Design review of the part shown in the three views and the two pictorial views. Dimensions are in mm from the part's minimum x, y and z. A direction names the side the tool comes from. Give positions to 0.01 mm unless a question says otherwise; leave off trailing zeros. Order: outer loops, then holes, each group sorted by start corner. A loop starts at its lowest first (then second) coordinate and runs counter-clockwise, first axis right, second up.
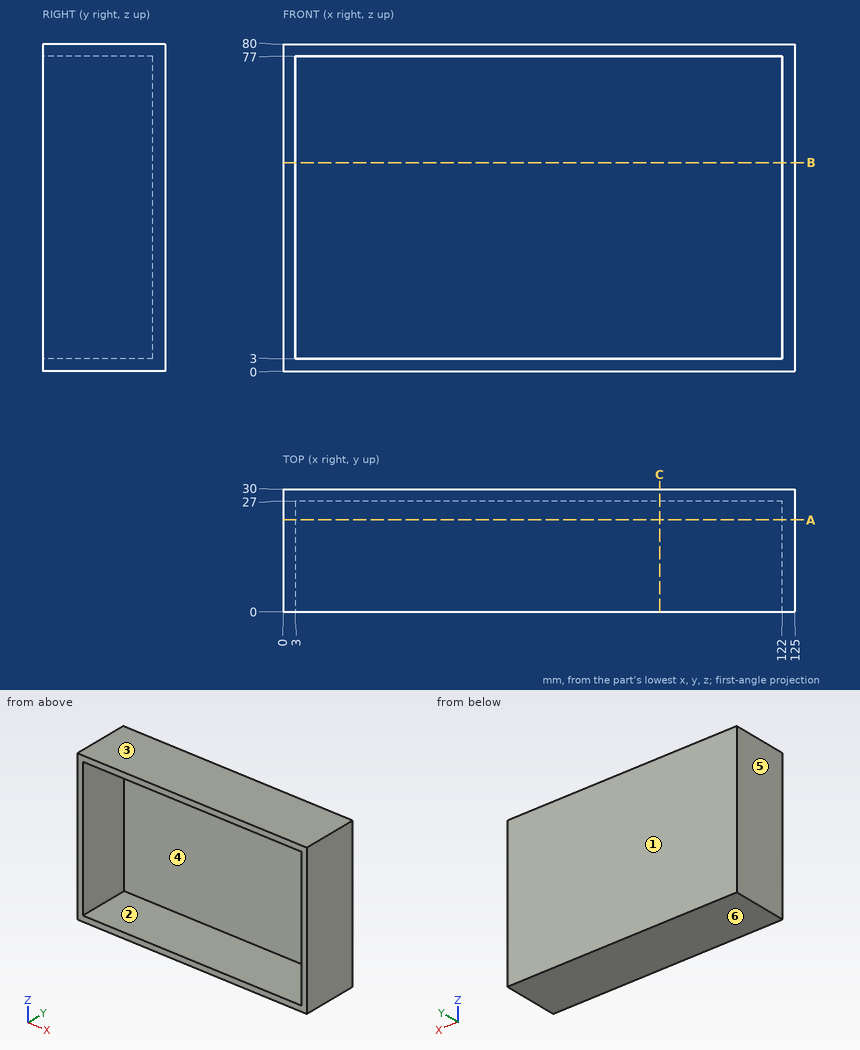
1) Tool access review of the marked faces 1 and 2: name each direction out of +Z, -Z, +X, -X, +Y, -Y from which nothing blocks a thin tool from reaching the whole face with its end or side.
Answer sheet:
face 1: +Z, -Z, +X, -X, +Y
face 2: -Y
2) Clearance check with flat-ended pins moving along their axes: pin 1 (5 mm diameter, centred on x = 51.5, z = 31, fed in from -Y); pin 2 (2 mm diameter, centred on x = 91.5, y = 23, fed in from -Z). State where each tip first meets the part, or that it passes through.
Answer sheet:
pin 1: stops at y = 27
pin 2: stops at z = 0
3) To check wall thickness, follow line 1 (Z direction, x = 71, y = 6.25); line 2 (X direction, y = 15, z = 38.5); line 3 (Y direction, x = 75, z = 40). State the ranges of each line that lie inside material, in increasing order.
Answer sheet:
line 1: z = 0 to 3, 77 to 80
line 2: x = 0 to 3, 122 to 125
line 3: y = 27 to 30
4) Draft analysis for pull direction Z (two halves, no side actions). For the marked faces 3, 4, 5 and 6, state which applies: +Z half, -Z half, draft (parallel to the pull), parting line (faces both ways), or undercut.
Answer sheet:
face 3: +Z half
face 4: undercut
face 5: draft
face 6: -Z half
5) We need section A-A on y = 22.5. Give the boundary of the cut face in (x, z), then the cut area to 3 significant figures.
Answer sheet:
outline: (0, 0) - (125, 0) - (125, 80) - (0, 80) - close; hole (3, 3) - (122, 3) - (122, 77) - (3, 77) - close
area: 1,190 mm2
6) We need section C-C on x = 92. Give the boundary of the cut face in (y, z).
Answer sheet:
outline: (0, 0) - (30, 0) - (30, 80) - (0, 80) - (0, 77) - (27, 77) - (27, 3) - (0, 3) - close
7) We need section B-B on z = 51. Give the boundary of the cut face in (x, y), then the cut area to 3 significant figures.
Answer sheet:
outline: (0, 0) - (3, 0) - (3, 27) - (122, 27) - (122, 0) - (125, 0) - (125, 30) - (0, 30) - close
area: 537 mm2
